Geometry: final body of the model. Coordinates: model frame, mm. A direction names the side the tool comes from. Coordinates: 2 decimals unless noted, no trailing zeros. Loops run counter-clockwise (first coordinate to the right, second up) from the corner with the lowest first, then second, coordinate; pieces in that order, holes last. Notation, with made-up numbers: (-2.5, -22) -> (37.5, -22) arc R17 ccw to (37.5, -4) -> close; hole circle Ø7 at (74, 8.25). An arc over 180 degrees is marked (long way). One line per item, written item: value. Start each with the question number.
Item 1: Ray query, probe 1 along X at (y, z) = (26.5, -1); probe 2 along X at (y, z) = (40, -43.5); probe 3 along Y at (x, z) = (56.5, 7). Return the intervals inside material, ascending. Write a range as from..to.
Item 2: Mould query, pull axis X, two halves, no side actions, for faces 5 (the cylindrical face through (15.096, 65.669, 54.374)), 6 (the flat face through (92.517, 6.162, 31.764)), 7 (the flat face through (73.515, 6.162, 64.095)), 8 (the flat face through (55, 68.75, -1)). Classes: +X half, -X half, draft (parallel to the pull), parting line (faces both ways), or undercut.
Item 3: Section query A-A on x = 0. Give the number of separate pieces and of enclosed holes in the cut face, then the cut area to 3 significant figures.
Item 4: Section query B-B on y = 6. Return loops of the section in (x, z) (3 decimals).
Item 5: Section query C-C on y = 23. Return loops of the section in (x, z).
Item 6: Contact query for flat-ended pins moving along their axis: pin 1 Ø2 at (x, y) = (27, 9) entering from -Z; pin 2 Ø7 at (y, z) = (65.5, -39.5) entering from -X; pin 3 Ø13.5 at (x, z) = (12.5, -43) entering from +Y. Output: stop coordinate, or through.
Item 7: Set-up query: faces 1 (the flat face through (34.375, 66, -1)), 2 (the flat face through (-18.75, 6, -96)), 3 (the flat face through (14, 62.5, 13)), 4 (the flat face through (82, 12.5, 54)). Return all of +Z, -Z, +X, -X, +Y, -Y with unobstructed straight access to the full face (end or side cutting, diameter ignored); none if empty.
from build123d import *

# Parameters (mm, degrees)
SKETCH1_R                = 87.5
BOSS_EXTRUDE1_DEPTH      = 68.75
FILLET1_R                = 25
SHELL1_T                 = -6.25
CUT_EXTRUDE1_DEPTH       = 68.75
BOSS_EXTRUDE2_DEPTH      = 12.75
BOSS_EXTRUDE2_DEPTH_BACK = 6.25
SKETCH3_R                = 31.25
SKETCH3_R_2              = 18.75
CUT_EXTRUDE2_START       = -12.75
SKETCH4_R                = 18.75
CUT_EXTRUDE2_DEPTH       = 12.75
SKETCH5_R                = 9
BOSS_EXTRUDE3_DEPTH      = 12.5


with BuildPart() as part:
    # Sketch1 → Boss-Extrude1 (new body)
    with BuildSketch(Plane(origin=(0, 0, 0), x_dir=(1, 0, 0), z_dir=(0, 1, 0))):
        with Locations(Location((0, 0, 0), (0, 0, 270))):
            Circle(SKETCH1_R)
    extrude(amount=BOSS_EXTRUDE1_DEPTH)

    # Fillet1
    fillet1_edges = [part.edges().sort_by_distance(p)[0] for p in [
        (0, 68.75, -87.5),
    ]]
    fillet(fillet1_edges, radius=FILLET1_R)

    # Shell1
    shell1_openings = [part.faces().sort_by_distance(p)[0] for p in [
        (0, 0, 0),
    ]]
    offset(amount=SHELL1_T, openings=shell1_openings, kind=Kind.INTERSECTION)

    # Sketch2 → Cut-Extrude1 (cut)
    with BuildSketch(Plane(origin=(0, 68.75, 0), x_dir=(1, 0, 0), z_dir=(0, 1, 0))):
        with BuildLine():
            Line((-34.375, -50), (-34.375, 50))
            ThreePointArc((-34.375, 50), (-30, 54.375), (-25.625, 50))
            Line((-25.625, 50), (-25.625, -50))
            ThreePointArc((-25.625, -50), (-30, -54.375), (-34.375, -50))
        make_face()
        with BuildLine():
            Line((-49.375, -50), (-49.375, 50))
            ThreePointArc((-49.375, 50), (-45, 54.375), (-40.625, 50))
            Line((-40.625, 50), (-40.625, -50))
            ThreePointArc((-40.625, -50), (-45, -54.375), (-49.375, -50))
        make_face()
        with BuildLine():
            Line((-19.375, -50), (-19.375, 50))
            ThreePointArc((-19.375, 50), (-15, 54.375), (-10.625, 50))
            Line((-10.625, 50), (-10.625, -50))
            ThreePointArc((-10.625, -50), (-15, -54.375), (-19.375, -50))
        make_face()
        with BuildLine():
            Line((-4.375, -50), (-4.375, 50))
            ThreePointArc((-4.375, 50), (0, 54.375), (4.375, 50))
            Line((4.375, 50), (4.375, -50))
            ThreePointArc((4.375, -50), (0, -54.375), (-4.375, -50))
        make_face()
        with BuildLine():
            Line((10.625, -50), (10.625, 50))
            ThreePointArc((10.625, 50), (15, 54.375), (19.375, 50))
            Line((19.375, 50), (19.375, -50))
            ThreePointArc((19.375, -50), (15, -54.375), (10.625, -50))
        make_face()
        with BuildLine():
            Line((25.625, -50), (25.625, 50))
            ThreePointArc((25.625, 50), (30, 54.375), (34.375, 50))
            Line((34.375, 50), (34.375, -50))
            ThreePointArc((34.375, -50), (30, -54.375), (25.625, -50))
        make_face()
        with BuildLine():
            Line((40.625, -50), (40.625, 50))
            ThreePointArc((40.625, 50), (45, 54.375), (49.375, 50))
            Line((49.375, 50), (49.375, -50))
            ThreePointArc((49.375, -50), (45, -54.375), (40.625, -50))
        make_face()
    extrude(amount=-CUT_EXTRUDE1_DEPTH, mode=Mode.SUBTRACT)

    # Sketch3 → Boss-Extrude2 (add, two sides: drawn at the far end of the back side and taken through both)
    with BuildSketch(Plane(origin=(0, 68.75, 0), x_dir=(1, 0, 0), z_dir=(0, 1, 0)).offset(-BOSS_EXTRUDE2_DEPTH_BACK)):
        with Locations(Location((0, 0, 0), (0, 0, 270))):
            Circle(SKETCH3_R)
        with Locations(Location((0, 0, 0), (0, 0, 270))):
            Circle(SKETCH3_R_2, mode=Mode.SUBTRACT)
    extrude(amount=BOSS_EXTRUDE2_DEPTH + BOSS_EXTRUDE2_DEPTH_BACK)

    # Sketch4 → Cut-Extrude2 (cut)
    with BuildSketch(Plane.XZ.offset(-62.5).offset(CUT_EXTRUDE2_START)):
        with Locations(Location((0, 0, 0), (0, 0, 90))):
            Circle(SKETCH4_R)
    extrude(amount=CUT_EXTRUDE2_DEPTH, mode=Mode.SUBTRACT)

    # Sketch5 → Boss-Extrude3 (add)
    # profile 1 of 3: a face of its own
    with BuildSketch(Plane(origin=(0, 0, 0), x_dir=(1, 0, 0), z_dir=(0, 1, 0))):
        with BuildLine():
            Line((-18.75, 106.25), (-18.75, 85.46746457))
            ThreePointArc((-18.75, 85.46746457), (0, 87.5), (18.75, 85.46746457))
            Line((18.75, 85.46746457), (18.75, 106.25))
            ThreePointArc((18.75, 106.25), (0, 125), (-18.75, 106.25))
        make_face()
        with Locations(Location((0, 106.25, 0), (0, 0, 270))):
            Circle(SKETCH5_R, mode=Mode.SUBTRACT)
    # profile 2 of 3: a face of its own
    with BuildSketch(Plane(origin=(0, 0, 0), x_dir=(1, 0, 0), z_dir=(0, 1, 0))):
        with BuildLine():
            Line((101.390199152, -36.887023679), (83.391995515, -26.495755964))
            ThreePointArc((83.391995515, -26.495755964), (75.777222831, -43.75), (64.641995515, -58.971708606))
            Line((64.641995515, -58.971708606), (82.640199152, -69.362976321))
            ThreePointArc((82.640199152, -69.362976321), (108.253175473, -62.5), (101.390199152, -36.887023679))
        make_face()
        with Locations(Location((92.015199152, -53.125, 0), (0, 0, 270))):
            Circle(SKETCH5_R, mode=Mode.SUBTRACT)
    # profile 3 of 3: a face of its own
    with BuildSketch(Plane(origin=(0, 0, 0), x_dir=(1, 0, 0), z_dir=(0, 1, 0))):
        with BuildLine():
            Line((-82.640199152, -69.362976321), (-64.641995515, -58.971708606))
            ThreePointArc((-64.641995515, -58.971708606), (-75.777222831, -43.75), (-83.391995515, -26.495755964))
            Line((-83.391995515, -26.495755964), (-101.390199152, -36.887023679))
            ThreePointArc((-101.390199152, -36.887023679), (-108.253175473, -62.5), (-82.640199152, -69.362976321))
        make_face()
        with Locations(Location((-92.015199152, -53.125, 0), (0, 0, 270))):
            Circle(SKETCH5_R, mode=Mode.SUBTRACT)
    extrude(amount=BOSS_EXTRUDE3_DEPTH)


solid = part.part
Reply:
1. probe 1: x = -87.49..-81.24, 81.24..87.49
1. probe 2: x = -75.92..-68.62, 68.62..75.92
1. probe 3: y = 62.5..68.75
2. face 5: undercut
2. face 6: +X half
2. face 7: undercut
2. face 8: draft
3. separate pieces: 5
3. enclosed holes: 0
3. area: 1,800 mm²
4. outline: (-101.39, 36.887) -> (-83.392, 26.496) arc R87.5 ccw to (-18.75, -85.467) -> (-18.75, -106.25) arc R18.75 ccw to (18.75, -106.25) -> (18.75, -85.467) arc R87.5 ccw to (83.392, 26.496) -> (101.39, 36.887) arc R18.75 ccw to (82.64, 69.363) -> (64.642, 58.972) arc R87.5 ccw to (-64.642, 58.972) -> (-82.64, 69.363) arc R18.75 ccw to start; hole circle Ø18 at (-92.015, 53.125); hole circle Ø162.5 at (0, 0); hole circle Ø18 at (0, -106.25); hole circle Ø18 at (92.015, 53.125)
5. outline: circle Ø175 at (0, 0); hole circle Ø162.5 at (0, 0)
6. pin 1: stops at z = -83.55
6. pin 2: stops at x = -69.51
6. pin 3: stops at y = 68.75
7. face 1: +Y, -Y
7. face 2: -Z, -X, +Y, -Y
7. face 3: -Y
7. face 4: +Z, +X, +Y
